Autodesk Inventor part; units mm, degrees
ref_plane "YZ Plane" through (0, 0, 0) normal (1, 0, 0) x (0, 1, 0)
ref_plane "XZ Plane" through (0, 0, 0) normal (0, 1, 0) x (-1, 0, 0)
ref_plane "XY Plane" through (0, 0, 0) normal (0, 0, 1) x (1, 0, 0)
sketch "Sketch1" plane through (0, 0, 0) normal (0, 1, 0) x (-1, 0, 0)
  line L0 (0, 0) -> (-196.85, 0)
  line L1 (-196.85, 0) -> (-196.85, 101.6)
  line L2 (-196.85, 101.6) -> (0, 101.6)
  line L3 (0, 101.6) -> (0, 0)
  dimension "d0" = 196.85
  dimension "d1" = 101.6
extrude "Plate1" add sketch "Sketch1" along normal blind 3.175
hole "Hole1" at (9.525, 3.175, 12.7) direction (0, -1, 0) diameter 6.35 end through all
hole "Hole2" at (187.325, 3.175, 12.7) direction (0, -1, 0) diameter 6.35 end through all
pattern_linear "Rectangular Pattern1" count 4 spacing 25.4 along (0, 0, 1) of "Hole1"
pattern_linear "Rectangular Pattern2" count 4 spacing 25.4 along (0, 0, 1) of "Hole2"
fillet "Fillet1" radius 6.35 1 edges at (0, 1.5875, 101.6)
fillet "Fillet2" radius 6.35 1 edges at (0, 1.5875, 0)
fillet "Fillet3" radius 6.35 1 edges at (196.85, 1.5875, 101.6)
fillet "Fillet4" radius 6.35 1 edges at (196.85, 1.5875, 0)
hole "Hole3" at (114.3, 3.175, 12.7) direction (0, -1, 0) diameter 6.35 end through all
pattern_linear "Rectangular Pattern3" count 2 spacing 76.2 along (0, 0, 1) of "Hole3"
equation "\"d10\" = Thickness"
equation "\"d19\" = Thickness"
equation "\"d38\" = Thickness"
equation "\"BendRadius\" = Thickness"
equation "\"BendReliefWidth\" = Thickness"
equation "\"BendReliefDepth\" = 0.5 * Thickness"
equation "\"CornerReliefSize\" = 4 * Thickness"
equation "\"MinimumRemnant\" = 2 * Thickness"
equation "\"TransitionRadius\" = BendRadius"
equation "\"JacobiRadiusSize\" = BendRadius"
equation "\"GapSize\" = Thickness"
equation "\"d2\" = BendRadius"
properties part number "Motor Mount"
Verification items for the finished model (mm, model axes). Give positions to 0.01 mm unless a question says otherwise; leave off trailing zeros. Order: outer loops, then holes, each group sorted by start corner. A loop starts at its lowest first (then second) coordinate and runs counter-clockwise, first axis right, second up. Notation, with made-up numbers: M -2,-10 L 43,-10 A25 cw 43,26 Z; hole C 30.25,-3.75 d8. An arc over 180 degrees is marked long. Answer as a JSON object with one key per item and string values. Group by question number.
1) Cross-section at D-D (y = 1.45). Give the number of separate pieces and of enclosed holes in the cut face, then the cut area to 3 significant figures.
2) Cross-section at C-C (z = 12.7). Enter the section's corners in (x, y) (3 decimals).
3) Scan lines: line 1 along X through (y, z) = (2.55, 38.1); line 2 along Z through (x, y) = (187.5, 1.7); line 3 along Z through (x, y) = (114.3, 0.85) (3 decimals). Record each from-to range of solid material in increasing order. Write a range as [from, to].
4) Mould release check, pull along Z, two halves, no side actions. Record for faces 1 (the face through (195.04, 1.61, 1.91)), 2 (the face through (184.177, 1.565, 37.687)), 3 (the face through (194.94, 1.61, 99.79)): released by +Z, released by -Z, zero draft, split by the parting line, or undercut.
5) Cross-section at B-B (z = 63.5). Enter the section's corners in (x, y) (3 decimals), then the cut area to 3 significant figures.
6) Cross-section at A-A (x = 114.3). Enter the section's corners in (y, z) (3 decimals).
Result sheet:
{
 "1": {"separate pieces": "1", "enclosed holes": "10", "area": "19,600 mm2"},
 "2": {"outline": "M 0,0 L 6.35,0 L 6.35,3.175 L 0,3.175 Z; M 12.7,0 L 111.125,0 L 111.125,3.175 L 12.7,3.175 Z; M 117.475,0 L 184.15,0 L 184.15,3.175 L 117.475,3.175 Z; M 190.5,0 L 196.85,0 L 196.85,3.175 L 190.5,3.175 Z"},
 "3": {"line 1": "x = [0, 6.35], [12.7, 184.15], [190.5, 196.85]", "line 2": "z = [0, 9.53], [15.87, 34.93], [41.27, 60.33], [66.67, 85.73], [92.07, 101.6]", "line 3": "z = [0, 9.525], [15.875, 85.725], [92.075, 101.6]"},
 "4": {"face 1": "released by -Z", "face 2": "undercut", "face 3": "released by +Z"},
 "5": {"outline": "M 0,0 L 6.35,0 L 6.35,3.175 L 0,3.175 Z; M 12.7,0 L 184.15,0 L 184.15,3.175 L 12.7,3.175 Z; M 190.5,0 L 196.85,0 L 196.85,3.175 L 190.5,3.175 Z", "area": "585 mm2"},
 "6": {"outline": "M 0,0 L 3.175,0 L 3.175,9.525 L 0,9.525 Z; M 0,15.875 L 3.175,15.875 L 3.175,85.725 L 0,85.725 Z; M 0,92.075 L 3.175,92.075 L 3.175,101.6 L 0,101.6 Z"}
}
